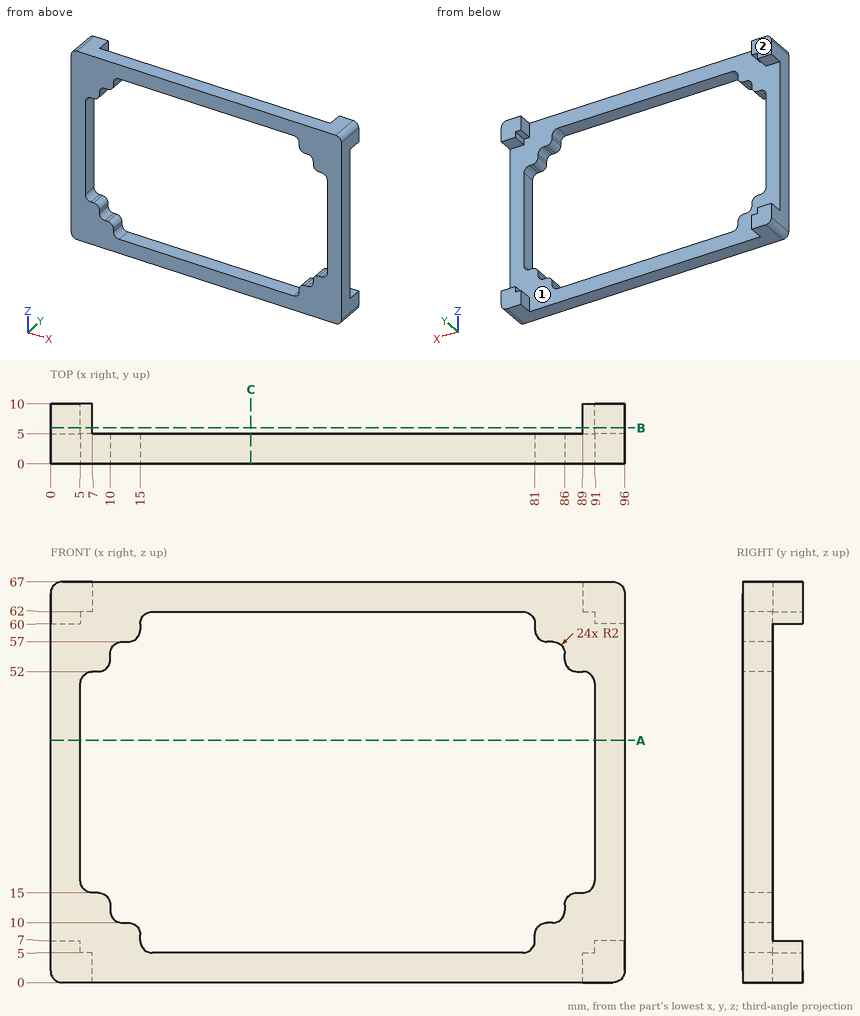
Geometry: see drawing. Coordinates: mm, zero at the bounding-box minimum. Round coordinates to 2 decimals unless told otherwise and drop trailing zeros. Write each loop counter-clockwise with the first axis right and the second up, starting at its lowest first coordinate (ties: lowest second). Pieces come first, ordered by that corner, then holes.
1) Cut plane A-A (z = 40.5). Return the cut outline in (x, y), then the cut area to 3 significant figures.
2) Cut plane B-B (y = 6). Return the cut outline in (x, z), then the cut area to 3 significant figures.
3) Cut plane C-C (x = 33.5). Return the cut outline in (y, z), then the cut area to 3 significant figures.
4) Draft query along X for the marked faces 1 and 2. Return one class per face: pulls with the +X half, pulls with the -X half, needs draft (parallel to the pull), parting line crosses it, or undercut.
5) Ray query, L1, parallel to X at y = 9.25, z = 62.5; L2, parallel to X at y = 4.25, z = 23; L3, parallel to Z at x = 62, y = 1.25. Return the intervals inside material, ascending.
6) Contact query for a flat-ended pin moving along its axis: P1, Ø4, axis at x = 60.5, y = 2.5, coming from the -Z side. Output: stop coordinate, or through.
Geometry says:
1. outline: (0, 0) - (5, 0) - (5, 5) - (0, 5) - close; (91, 0) - (96, 0) - (96, 5) - (91, 5) - close
1. area: 50.0 mm2
2. outline: (0, 2) arc R2 ccw to (2, 0) - (7, 0) - (7, 5) - (5, 5) - (5, 7) - (0, 7) - close; (0, 60) - (5, 60) - (5, 62) - (7, 62) - (7, 67) - (2, 67) arc R2 ccw to (0, 65) - close; (89, 0) - (94, 0) arc R2 ccw to (96, 2) - (96, 7) - (91, 7) - (91, 5) - (89, 5) - close; (89, 62) - (91, 62) - (91, 60) - (96, 60) - (96, 65) arc R2 ccw to (94, 67) - (89, 67) - close
2. area: 177 mm2
3. outline: (0, 0) - (5, 0) - (5, 5) - (0, 5) - close; (0, 62) - (5, 62) - (5, 67) - (0, 67) - close
3. area: 50.0 mm2
4. face 1: undercut
4. face 2: needs draft
5. L1: x = 0 to 7, 89 to 96
5. L2: x = 0 to 5, 91 to 96
5. L3: z = 0 to 5, 62 to 67
6. P1: stops at z = 0
